```python
from build123d import *

# Parameters (mm, degrees)
SKETCH1_R           = 15
BOSS_EXTRUDE1_DEPTH = 5
SKETCH2_R           = 5
BOSS_EXTRUDE2_DEPTH = 89
CUT_EXTRUDE2_START  = -10
CUT_EXTRUDE2_DEPTH  = 10
CIRPATTERN1_COUNT   = 3


with BuildPart() as part:
    # Sketch1 → Boss-Extrude1 (new body)
    with BuildSketch(Plane(origin=(0, 0, 0), x_dir=(1, 0, 0), z_dir=(0, 1, 0))):
        with Locations(Location((0, 0, 0), (0, 0, 270))):
            Circle(SKETCH1_R)
    extrude(amount=-BOSS_EXTRUDE1_DEPTH)

    # Sketch2 → Boss-Extrude2 (add)
    with BuildSketch(Plane(origin=(0, 0, 0), x_dir=(1, 0, 0), z_dir=(0, 1, 0))):
        with Locations(Location((0, 0, 0), (0, 0, 270))):
            Circle(SKETCH2_R)
    extrude(amount=BOSS_EXTRUDE2_DEPTH)

    # Sketch7 → Cut-Extrude2 (cut)
    with BuildSketch(Plane(origin=(0, 89, 0), x_dir=(1, 0, 0), z_dir=(0, 1, 0)).offset(CUT_EXTRUDE2_START)):
        with BuildLine():
            Line((-1.5612495, 4.75), (1.5612495, 4.75))
            ThreePointArc((1.5612495, 4.75), (0, 5), (-1.5612495, 4.75))
        make_face()
    cut_extrude2 = extrude(amount=CUT_EXTRUDE2_DEPTH, mode=Mode.SUBTRACT)

    # CirPattern1: Cut-Extrude2 ×3 about axis
    cirpattern1_axis = Axis((0, 0, 0), (0, 1, 0))
    for i in range(1, CIRPATTERN1_COUNT):
        add(cut_extrude2.rotate(cirpattern1_axis, i * 360 / CIRPATTERN1_COUNT), mode=Mode.SUBTRACT)


solid = part.part
```
The listing builds one solid part. Answer for the finished solid, in the listing's coordinates (mm). A direction names the side the tool comes from. Round coordinates to 2 decimals unless told otherwise and drop trailing zeros. Loops run counter-clockwise (first coordinate to the right, second up) from the corner with the lowest first, then second, coordinate; pieces in that order, holes last. Notation, with made-up numbers: (17.25, 51.5) - (42.25, 51.5) arc R28 ccw to (42.25, 77.5) - close; hole circle Ø9 at (4, 51.25). An arc over 180 degrees is marked (long way). Return JSON: item names as keys, results as strings. Group by question number.
1. The part is cut by section C-C on y = 14.5. Determine the outline of the cut face in (x, z).
2. The part is cut by section D-D on z = -11.75. Determine the outline of the cut face in (x, y).
3. Which of the six approach directions +Z, -Z, +X, -X, +Y, -Y give full straight-line access (tool end or side, diameter ignored) to faces 1 (the flat face through (4, 0, -4)), 2 (the flat face through (0, 84, -4.75)), 3 (the flat face through (4.1, 83.9, 2.4)), 4 (the flat face through (-4.1, 83.9, 2.4))?
4. Consider probe 1 along Y at (x, z) = (-3.5, -7); probe 2 along Z at (x, y) = (-1, 70); probe 3 along X at (y, z) = (59.5, 0). Determine where each line is inside the solid, lowest interval first.
5. Each of these flat-tipped pins is pushed along its axis until it touches: P1, Ø1, axis at y = 40, z = -3, coming from the +X side; P2, Ø12, axis at x = 1.5, y = 55.5, coming from the +Z side; P3, Ø4, axis at x = -1.5, y = 54.5, coming from the -Z side. Where does it stop, or does it pass through?
6. The part is cut by section A-A on x = 0. Determine the outline of the cut face in (y, z), then the cut area to 3 significant figures.
7. The part is cut by section B-B on z = 0. Determine the outline of the cut face in (x, y), then the cut area to 3 significant figures.
Resolved:
{
 "1": {"outline": "circle Ø10 at (0, 0)"},
 "2": {"outline": "(-9.32, -5) - (9.32, -5) - (9.32, 0) - (-9.32, 0) - close"},
 "3": {"face 1": "+Y", "face 2": "-Z, +X, -X, +Y", "face 3": "+Z, +X, +Y", "face 4": "+Z, -X, +Y"},
 "4": {"probe 1": "y = -5 to 0", "probe 2": "z = -4.9 to 4.9", "probe 3": "x = -5 to 5"},
 "5": {"P1": "stops at x = 4.33", "P2": "stops at z = 5", "P3": "stops at z = -5"},
 "6": {"outline": "(-5, -15) - (0, -15) - (0, -5) - (79, -5) - (79, -4.75) - (89, -4.75) - (89, 5) - (0, 5) - (0, 15) - (-5, 15) - close", "area": "1,040 mm²"},
 "7": {"outline": "(-15, -5) - (15, -5) - (15, 0) - (5, 0) - (5, 89) - (-5, 89) - (-5, 0) - (-15, 0) - close", "area": "1,040 mm²"}
}
